Input: dimensioned drawing with shaded views. Units: mm. Origin: part minimum x, y, z. Coordinates: 2 decimals unless noted, no trailing zeros. Write item = value, one per line. Start each with the question number.
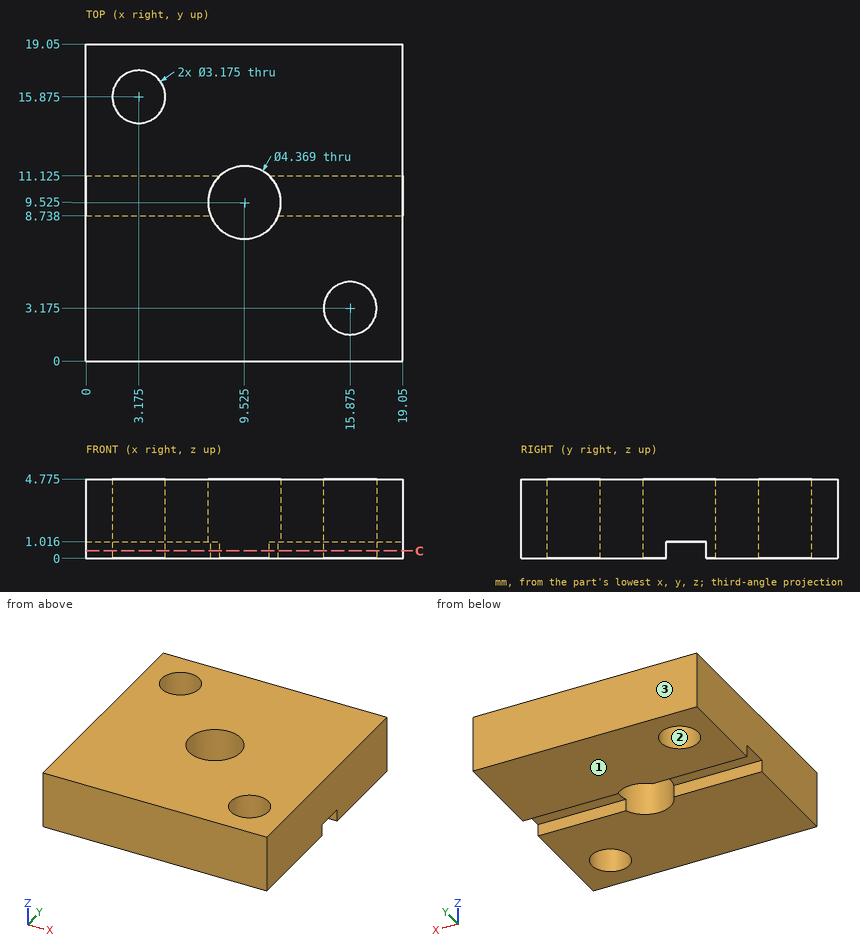
Item 1: Section query C-C (z = 0.45). Count the separate pieces of the cut face and the enclosed holes in it, plus the area to 3 significant figures.
Item 2: Pull-direction query (Y, two-part tool) for the marked faces 1, 2 and 3; classes: released by +Y, released by -Y, zero draft, split by the parting line, or undercut.
Item 3: Line query: line 1 (X direction, y = 16, z = 0.5); line 2 (Y direction, x = 8.75, z = 0.6); line 3 (Y direction, x = 4.5, z = 2.85). Output: solid intervals per line, ascending. Write a range as from..to.
Item 4: First-contact query: pin 1 (5 mm diameter, centred on x = 3.175, y = 15.875, fed in from -Z); pin 2 (1.2 mm diameter, centred on x = 16.5, y = 9.5, fed in from -Z); pin 3 (3.5 mm diameter, centred on x = 9.525, y = 9.525, fed in from +Z). Flat tips, straight axial feed; report the tip coordinate or a pass-through.
Verdict:
q1.separate_pieces = 2
q1.enclosed_holes = 2
q1.area = 296 mm2
q2.face_1 = zero draft
q2.face_2 = undercut
q2.face_3 = released by +Y
q3.line_1 = 0..1.59, 4.76..19.05
q3.line_2 = 0..7.48, 11.57..19.05
q3.line_3 = 0..15, 16.75..19.05
q4.pin_1 = 0
q4.pin_2 = 1.02
q4.pin_3 = through
